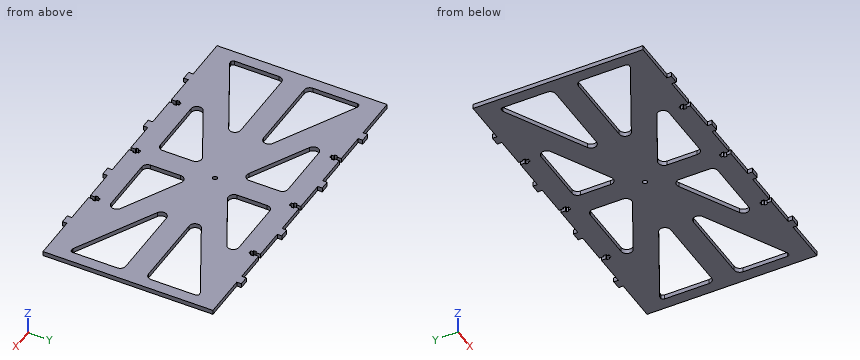
from build123d import *

# Parameters (mm, degrees)
EXTRUDE_1_DEPTH     = 4
SKETCH_4_R          = 2
CUT_EXTRUDE_1_DEPTH = 10


with BuildPart() as part:
    # 草图1 → 凸台-拉伸1 (new body)
    with BuildSketch(Plane.XY):
        Polygon((0, -4), (0, 0), (-27.5, 0), (-27.5, 4), (-35.5, 4), (-35.5, 0), (-63, 0), (-63, -4), (-61.65, -4), (-61.65, -6.6), (-63, -6.6), (-63, -8.6), (-66, -8.6), (-66, -6.6), (-67.35, -6.6), (-67.35, -4), (-66, -4), (-66, 0), (-93.5, 0), (-93.5, 4), (-101.5, 4), (-101.5, 0), (-129, 0), (-140.5, 0), (-140.5, -150), (-129, -150), (-101.5, -150), (-101.5, -154), (-93.5, -154), (-93.5, -150), (-66, -150), (-66, -146), (-67.35, -146), (-67.35, -143.4), (-66, -143.4), (-66, -141.4), (-63, -141.4), (-63, -143.4), (-61.65, -143.4), (-61.65, -146), (-63, -146), (-63, -150), (-35.5, -150), (-35.5, -154), (-27.5, -154), (-27.5, -150), (0, -150), (0, -146), (-1.35, -146), (-1.35, -143.4), (0, -143.4), (0, -141.4), (3, -141.4), (3, -143.4), (4.35, -143.4), (4.35, -146), (3, -146), (3, -150), (30.5, -150), (30.5, -154), (38.5, -154), (38.5, -150), (66, -150), (66, -146), (64.65, -146), (64.65, -143.4), (66, -143.4), (66, -141.4), (69, -141.4), (69, -143.4), (70.35, -143.4), (70.35, -146), (69, -146), (69, -150), (96.5, -150), (96.5, -154), (104.5, -154), (104.5, -150), (132, -150), (143.5, -150), (143.5, 0), (132, 0), (104.5, 0), (104.5, 4), (96.5, 4), (96.5, 0), (69, 0), (69, -4), (70.35, -4), (70.35, -6.6), (69, -6.6), (69, -8.6), (66, -8.6), (66, -6.6), (64.65, -6.6), (64.65, -4), (66, -4), (66, 0), (38.5, 0), (38.5, 4), (30.5, 4), (30.5, 0), (3, 0), (3, -4), (4.35, -4), (4.35, -6.6), (3, -6.6), (3, -8.6), (0, -8.6), (0, -6.6), (-1.35, -6.6), (-1.35, -4), align=None)
    extrude(amount=EXTRUDE_1_DEPTH)

    # 草图4 → 切除-拉伸1 (cut)
    with BuildSketch(Plane.XY.offset(4)):
        with BuildLine():
            ThreePointArc((-127.191659555, -18.6), (-126.710498265, -18.658741693), (-126.257601204, -18.831516187))
            Line((-126.257601204, -18.831516187), (-56.682761898, -55.578790468))
            ThreePointArc((-56.682761898, -55.578790468), (-54.164762011, -61.202903226), (-59.017907777, -65))
            Line((-59.017907777, -65), (-125.5, -65))
            ThreePointArc((-125.5, -65), (-129.035533906, -63.535533906), (-130.5, -60))
            Line((-130.5, -60), (-130.5, -20.6))
            ThreePointArc((-130.5, -20.6), (-129.914213562, -19.185786438), (-128.5, -18.6))
            Line((-128.5, -18.6), (-127.191659555, -18.6))
        make_face()
        with BuildLine():
            ThreePointArc((-130.5, -90), (-129.035533906, -86.464466094), (-125.5, -85))
            Line((-125.5, -85), (-59.017907777, -85))
            ThreePointArc((-59.017907777, -85), (-54.164762011, -88.797096774), (-56.682761898, -94.421209532))
            Line((-56.682761898, -94.421209532), (-126.257601204, -131.168483813))
            ThreePointArc((-126.257601204, -131.168483813), (-126.710498265, -131.341258307), (-127.191659555, -131.4))
            Line((-127.191659555, -131.4), (-128.5, -131.4))
            ThreePointArc((-128.5, -131.4), (-129.914213562, -130.814213562), (-130.5, -129.4))
            Line((-130.5, -129.4), (-130.5, -90))
        make_face()
        with BuildLine():
            Line((-15.835145879, -95.465009365), (-66.034571435, -121.978790468))
            ThreePointArc((-66.034571435, -121.978790468), (-68.552571322, -127.602903226), (-63.699425556, -131.4))
            Line((-63.699425556, -131.4), (-13.5, -131.4))
            ThreePointArc((-13.5, -131.4), (-9.964466094, -129.935533906), (-8.5, -126.4))
            Line((-8.5, -126.4), (-8.5, -99.886218897))
            ThreePointArc((-8.5, -99.886218897), (-10.918888747, -95.603945587), (-15.835145879, -95.465009365))
        make_face()
        with BuildLine():
            Line((18.835145879, -95.465009365), (69.034571435, -121.978790468))
            ThreePointArc((69.034571435, -121.978790468), (71.552571322, -127.602903226), (66.699425556, -131.4))
            Line((66.699425556, -131.4), (16.5, -131.4))
            ThreePointArc((16.5, -131.4), (12.964466094, -129.935533906), (11.5, -126.4))
            Line((11.5, -126.4), (11.5, -99.886218897))
            ThreePointArc((11.5, -99.886218897), (13.918888747, -95.603945587), (18.835145879, -95.465009365))
        make_face()
        with BuildLine():
            ThreePointArc((130.191659555, -131.4), (129.710498265, -131.341258307), (129.257601204, -131.168483813))
            Line((129.257601204, -131.168483813), (59.682761898, -94.421209532))
            ThreePointArc((59.682761898, -94.421209532), (57.164762011, -88.797096774), (62.017907777, -85))
            Line((62.017907777, -85), (128.5, -85))
            ThreePointArc((128.5, -85), (132.035533906, -86.464466094), (133.5, -90))
            Line((133.5, -90), (133.5, -129.4))
            ThreePointArc((133.5, -129.4), (132.914213562, -130.814213562), (131.5, -131.4))
            Line((131.5, -131.4), (130.191659555, -131.4))
        make_face()
        with BuildLine():
            ThreePointArc((133.5, -60), (132.035533906, -63.535533906), (128.5, -65))
            Line((128.5, -65), (62.017907777, -65))
            ThreePointArc((62.017907777, -65), (57.164762011, -61.202903226), (59.682761898, -55.578790468))
            Line((59.682761898, -55.578790468), (129.257601204, -18.831516187))
            ThreePointArc((129.257601204, -18.831516187), (129.710498265, -18.658741693), (130.191659555, -18.6))
            Line((130.191659555, -18.6), (131.5, -18.6))
            ThreePointArc((131.5, -18.6), (132.914213562, -19.185786438), (133.5, -20.6))
            Line((133.5, -20.6), (133.5, -60))
        make_face()
        with BuildLine():
            Line((18.835145879, -54.534990635), (69.034571435, -28.021209532))
            ThreePointArc((69.034571435, -28.021209532), (71.552571322, -22.397096774), (66.699425556, -18.6))
            Line((66.699425556, -18.6), (16.5, -18.6))
            ThreePointArc((16.5, -18.6), (12.964466094, -20.064466094), (11.5, -23.6))
            Line((11.5, -23.6), (11.5, -50.113781103))
            ThreePointArc((11.5, -50.113781103), (13.918888747, -54.396054413), (18.835145879, -54.534990635))
        make_face()
        with BuildLine():
            Line((-15.835145879, -54.534990635), (-66.034571435, -28.021209532))
            ThreePointArc((-66.034571435, -28.021209532), (-68.552571322, -22.397096774), (-63.699425556, -18.6))
            Line((-63.699425556, -18.6), (-13.5, -18.6))
            ThreePointArc((-13.5, -18.6), (-9.964466094, -20.064466094), (-8.5, -23.6))
            Line((-8.5, -23.6), (-8.5, -50.113781103))
            ThreePointArc((-8.5, -50.113781103), (-10.918888747, -54.396054413), (-15.835145879, -54.534990635))
        make_face()
        with Locations((1.5, -75)):
            Circle(SKETCH_4_R)
    extrude(amount=-CUT_EXTRUDE_1_DEPTH, mode=Mode.SUBTRACT)


solid = part.part
For this review, take the finished solid that the model builds, in its own axes (mm). Coordinates: 2 decimals unless noted, no trailing zeros. Write each loop counter-clockwise with the first axis right and the second up, starting at its lowest first coordinate (ties: lowest second). Pieces come first, ordered by that corner, then holes. Notation, with made-up numbers: (86.25, 11.25) -> (125.25, 11.25) arc R22 cw to (125.25, 28.25) -> close; hole circle Ø7 at (14, 31). An arc over 180 degrees is marked (long way). Write each question's results on one line, items separated by ' | '. Start each with the question number.
1) Insertion check: pin 1 (1.2 mm diameter, centred on x = -83.5, z = 1.5, fed in from +Y); pin 2 (2 mm diameter, centred on x = 15.5, z = 2, fed in from -Y); pin 3 (10 mm diameter, centred on x = -15, y = -118.5, fed in from +Z) (1 decimal). Each pin has a flat end and moves straight along its axis. Give the tip position at first contact, or say it passes through.
2) Consider section A-A (x = -89.5). Write out the cut boundary in (y, z), plus the area to 3 significant figures.
3) Wall thickness on L1, parallel to Y at x = 1.5, z = 2.7; L2, parallel to Y at x = -32.5, z = 1.3; L3, parallel to X at y = -104, z = 1.5: over which ranges is each line inside the solid? List them lowest first. Write a range as [from, to].
4) Consider section C-C (x = -4.5). Write out the cut boundary in (y, z), plus the area to 3 significant figures.
5) Consider section B-B (z = 1.9). Give the number of separate pieces and of enclosed holes in the cut face, plus the area to 3 significant figures.
Geometry says:
1) pin 1: y = 0 | pin 2: y = -150 | pin 3: through
2) outline: (-150, 0) -> (-111.75, 0) -> (-111.75, 4) -> (-150, 4) -> close; (-85, 0) -> (-65, 0) -> (-65, 4) -> (-85, 4) -> close; (-38.25, 0) -> (0, 0) -> (0, 4) -> (-38.25, 4) -> close | area: 386 mm^2
3) L1: [-141.4, -77], [-73, -8.6] | L2: [-154, -131.4], [-104.27, -45.73], [-18.6, 4] | L3: [-140.5, -130.5], [-74.82, -31.99], [-8.5, 11.5], [34.99, 77.82], [133.5, 143.5]
4) outline: (-150, 0) -> (0, 0) -> (0, 4) -> (-150, 4) -> close | area: 600 mm^2
5) separate pieces: 1 | enclosed holes: 9 | area: 28,400 mm^2
